Design review of the part shown in the three views and the two pictorial views. Dimensions are in mm from the part's minimum x, y and z. A direction names the side the tool comes from. Coordinates: 2 decimals unless noted, no trailing zeros. Write each loop counter-clockwise with the first axis right and the second up, starting at its lowest first coordinate (ties: lowest second). Pieces come first, ordered by that corner, then holes.
Q1. For pin 1 Ø12 at (y, z) = (660, 36) entering from -X; pin 2 Ø10 at (x, z) = (35.5, 28) entering from +Y; pin 3 Ø3 at (x, z) = (140.5, 35.5) entering from +Y, all flat-tipped, find the tip position at first contact; note any pin that passes through.
Q2. Take a section at B-B, the plane y = 274.5. Write out the cut boundary in (x, z), plus the area to 3 significant figures.
Q3. Take a section at C-C, the plane x = 141. Write out the cut boundary in (y, z).
Q4. Take a section at A-A, the plane z = 31. Write out the cut boundary in (x, y).
Q5. The part is to be moulded in two halves that separate along X. For the marked faces 4, 5, 6 and 7, say which applies: released by +X, released by -X, zero draft, split by the parting line, or undercut.
Q6. For L1, parallel to X at y = 153, z = 14; L2, parallel to X at y = 54, z = 38; L3, parallel to Y at x = 10.5, z = 24.5, list the stretches that pass through material, from the lowest coordinate up.
Q7. For the marked faces 1, 2 and 3, list the 3-axis set-ups (+Z, -Z, +X, -X, +Y, -Y) from which the entire face can be reached by the end or side of a thin tool; tool diameter is ignored.
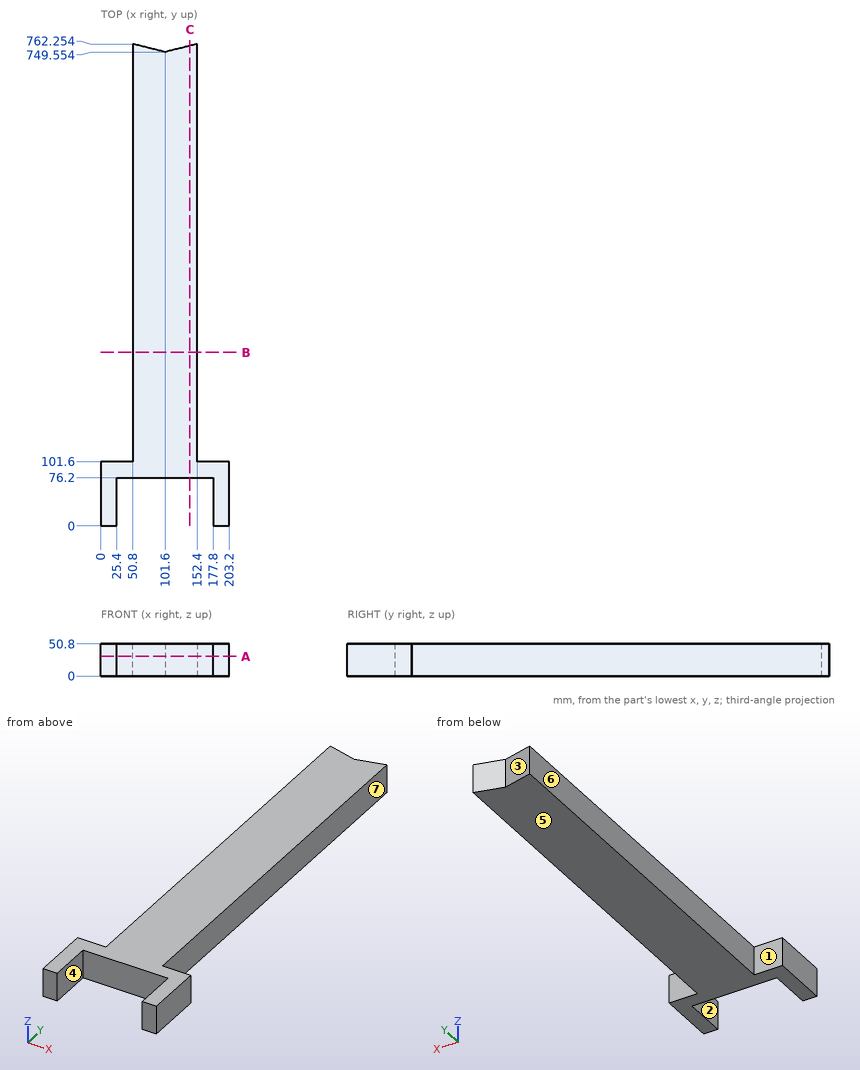
Responses:
1. pin 1: stops at x = 50.8
1. pin 2: stops at y = 101.6
1. pin 3: stops at y = 759.65
2. outline: (50.8, 0) - (152.4, 0) - (152.4, 50.8) - (50.8, 50.8) - close
2. area: 5,160 mm2
3. outline: (76.2, 0) - (759.4, 0) - (759.4, 50.8) - (76.2, 50.8) - close
4. outline: (0, 0) - (25.4, 0) - (25.4, 76.2) - (177.8, 76.2) - (177.8, 0) - (203.2, 0) - (203.2, 101.6) - (152.4, 101.6) - (152.4, 762.25) - (101.6, 749.55) - (50.8, 762.25) - (50.8, 101.6) - (0, 101.6) - close
5. face 4: undercut
5. face 5: zero draft
5. face 6: released by -X
5. face 7: released by +X
6. L1: x = 50.8 to 152.4
6. L2: x = 0 to 25.4, 177.8 to 203.2
6. L3: y = 0 to 101.6
7. face 1: +Z, -Z, -X, +Y
7. face 2: +Z, -Z, -Y
7. face 3: +Z, -Z, +Y
